Check sheet for the drawn part. Datum: minimum x, y, z corner. Units: mm. A direction names the side the tool comes from. Give positions to 0.01 mm unless a question says otherwise; leave off trailing zeros. Write each loop counter-clockwise with the first axis right and the second up, starting at its lowest first coordinate (ties: lowest second). Pieces come first, ordered by that corner, then holes. Notation, with made-up numbers: (33.5, 32) -> (51.5, 32) arc R10 cw to (51.5, 41) -> close; hole circle Ø2 at (39, 11.5). An arc over 180 degrees is marked (long way). Answer as CSV lines item,"result". Start each with the question number.
1) Sectioned sample at C-C on z = 1.9. Record the cut outline in (x, y).
2) Gauge pin test, flat ends, axial feed: pin 1 Ø5 at (x, y) = (5.5, 24.5) entering from +Z; pin 2 Ø2.5 at (x, y) = (16, 8.03) entering from -Z; pin 3 Ø0.6 at (x, z) = (16, 0.5) entering from -Y; pin 4 Ø1.2 at (x, z) = (14, 4) entering from -Y. Record the tip position at first contact, or that the pin passes through.
3) Sectioned sample at B-B on y = 20. Record the cut outline in (x, z).
4) Tool access check on the marked faces 1, 2 and 3. Record the directions out of +Z, -Z, +X, -X, +Y, -Y that give a thin tool (end or side, any length) a straight path to the whole face; none if there is none.
5) Material ranges on L1, parallel to Y at x = 10, z = 2.05; L2, parallel to Y at x = 15, z = 2.05; L3, parallel to Z at x = 2, y = 24, recorded low to high.
6) Sectioned sample at D-D on x = 8.5. Record the cut outline in (y, z) (3 decimals), and give its area (3 significant figures).
7) Sectioned sample at A-A on x = 19.5. Record the cut outline in (y, z), and give its area (3 significant figures).
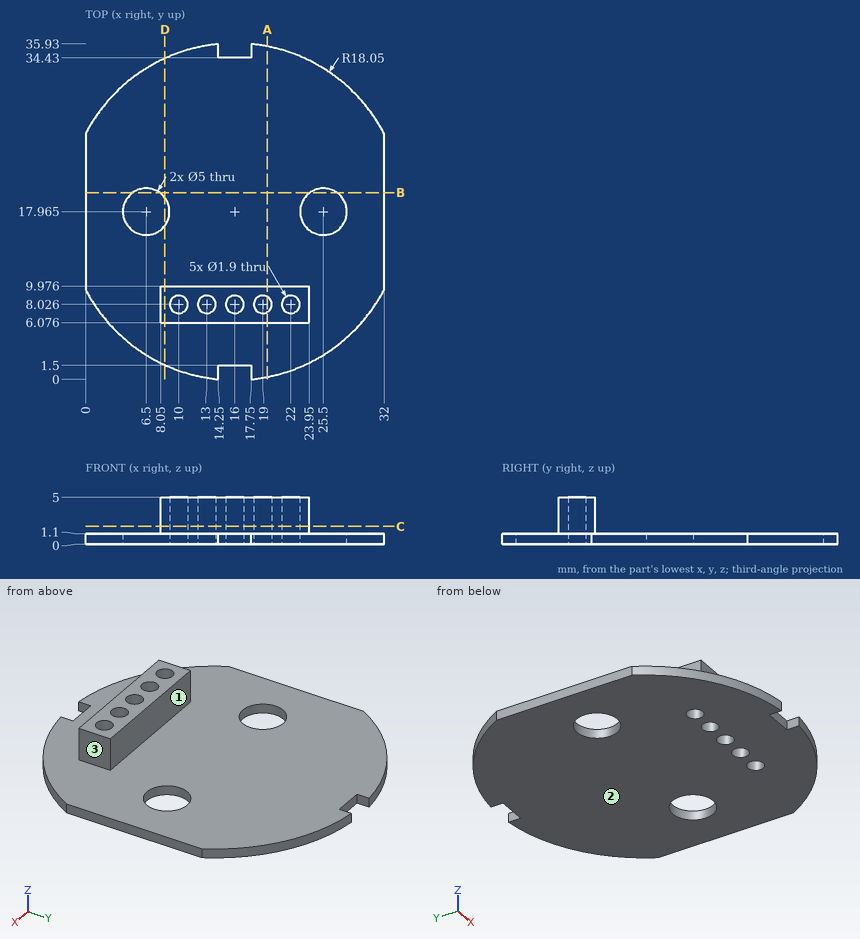
Ans:
1,outline,"(8.05, 6.08) -> (23.95, 6.08) -> (23.95, 9.98) -> (8.05, 9.98) -> close; hole circle Ø1.9 at (10, 8.03); hole circle Ø1.9 at (13, 8.03); hole circle Ø1.9 at (16, 8.03); hole circle Ø1.9 at (19, 8.03); hole circle Ø1.9 at (22, 8.03)"
2,pin 1,"stops at z = 1.1"
2,pin 2,"stops at z = 0"
2,pin 3,"stops at y = 1.5"
2,pin 4,"stops at y = 6.08"
3,outline,"(0, 0) -> (5.05, 0) -> (5.05, 1.1) -> (0, 1.1) -> close; (7.95, 0) -> (24.05, 0) -> (24.05, 1.1) -> (7.95, 1.1) -> close; (26.95, 0) -> (32, 0) -> (32, 1.1) -> (26.95, 1.1) -> close"
4,face 1,"+Z, +X, -X, +Y"
4,face 2,"-Z, +X, -X, +Y, -Y"
4,face 3,"+Z, +X, +Y, -Y"
5,L1,"y = 6.08 to 7.08, 8.98 to 9.98"
5,L2,"y = 6.08 to 9.98"
5,L3,"z = 0 to 1.1"
6,outline,"(1.547, 0) -> (16.465, 0) -> (16.465, 1.1) -> (9.976, 1.1) -> (9.976, 5) -> (6.076, 5) -> (6.076, 1.1) -> (1.547, 1.1) -> close; (19.465, 0) -> (34.383, 0) -> (34.383, 1.1) -> (19.465, 1.1) -> close"
6,area,"48.0 mm²"
7,outline,"(0.26, 0) -> (7.22, 0) -> (7.22, 5) -> (6.08, 5) -> (6.08, 1.1) -> (0.26, 1.1) -> close; (8.83, 0) -> (35.67, 0) -> (35.67, 1.1) -> (9.98, 1.1) -> (9.98, 5) -> (8.83, 5) -> close"
7,area,"46.1 mm²"
